```python
from build123d import *

# Parameters (mm, degrees)
F0_W      = 80
F0_H      = 30
F1_DEPTH  = 25
F3_DEPTH  = 20
F4_R      = 1.5
F5_DEPTH  = 1000
F3_FACE_W = 60.621056
F3_FACE_H = 22.732896
F6_DEPTH  = 25
F7_R      = 1.35
F7_R_2    = 1
F8_DEPTH  = 100000


with BuildPart() as f1:
    # F0 (on Front) → F1 (new body)
    with BuildSketch(Plane.XZ):
        with Locations((5.157232, 15)):
            Rectangle(F0_W, F0_H)
    extrude(amount=F1_DEPTH)

    # F2 (on face) → F3 (cut)
    with BuildSketch(Plane.XZ.offset(25)):
        Polygon((35.46776, 26.366448), (-25.153296, 26.366448), (5.157232, 15), align=None)
        Polygon((5.157232, 15), (-25.153296, 26.366448), (-25.153296, 3.633552), align=None)
        Polygon((35.46776, 26.366448), (5.157232, 15), (35.46776, 3.633552), align=None)
        Polygon((35.46776, 3.633552), (5.157232, 15), (-25.153296, 3.633552), align=None)
    extrude(amount=-F3_DEPTH, mode=Mode.SUBTRACT)

    # F4 (on face) → F5 (cut)
    with BuildSketch(Plane.YZ.offset(45.157232)):
        with Locations((-12.5, 15.157233)):
            Circle(F4_R)
    extrude(amount=-F5_DEPTH, mode=Mode.SUBTRACT)

    # F3_face (on face) → F6 (cut)
    with BuildSketch(Plane(origin=(5.157232, -5, 15), x_dir=(1, 0, 0), z_dir=(0, -1, 0))):
        Rectangle(F3_FACE_W, F3_FACE_H)
    extrude(amount=-F6_DEPTH, mode=Mode.SUBTRACT)

    # F7 (on face) → F8 (cut)
    with BuildSketch(Plane.XZ.offset(25)):
        with BuildLine():
            ThreePointArc((-29.95245, 20.807233), (-28.997856, 21.202639), (-28.60245, 22.157233))
            ThreePointArc((-28.60245, 22.157233), (-30.907045, 23.111827), (-29.95245, 20.807233))
        make_face()
        with Locations((-29.95245, 8.157233)):
            Circle(F7_R)
        with Locations((40.266914, 8.157233)):
            Circle(F7_R)
        with Locations((40.266914, 22.157233)):
            Circle(F7_R)
        with Locations((-12.661189, -18.048356)):
            Circle(F7_R_2)
    extrude(amount=-F8_DEPTH, mode=Mode.SUBTRACT)


solid = f1.part
```
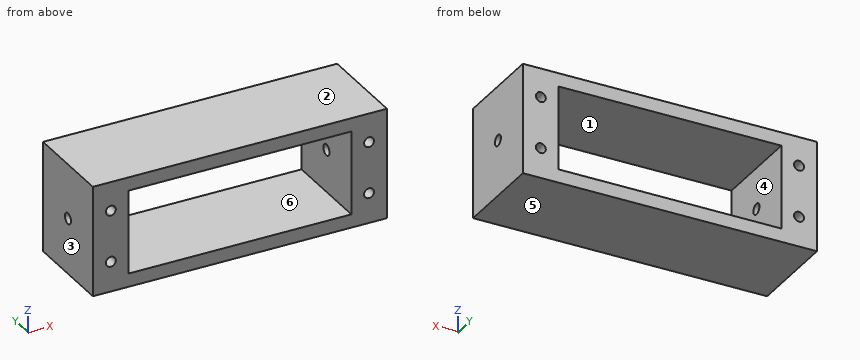
Can you work these out from the model? Positions are in its coordinate system, mm. Face numbers are marked on the shaded views. A direction names the side the tool comes from. Round coordinates to 2 decimals unless told otherwise and drop trailing zeros. Loops run counter-clockwise (first coordinate to the right, second up) from the corner with the lowest first, then second, coordinate; pieces in that order, holes last. Notation, with made-up numbers: M 22.25,88.5 L 48.25,88.5 A20 ccw 48.25,102.5 Z; hole C -22.5,47.5 d7. An arc over 180 degrees is marked long. Write item = value, one per line. Start each with the question number.
(1) I'm going to push a flat-ended pin straight in: P1, Ø2.5, axis at y = -12.5, z = 15.16, coming from the +X side. Where does the tip first touch, or does it pass through?
(2) If we mould it in two halves opening along X, with no side actions, what happens to the marked faces 1, 2, 3 and 4? For each: released by +X, released by -X, zero draft, split by the parting line, or undercut.
(3) Which directions (+Z, -Z, +X, -X, +Y, -Y) give clear straight access to the entire face, cutting with the end or side of a thin tool? Please do the marked faces 5 and 6.
(4) Suppose I cut it at C-C on x = 31.5. Write out the boundary of the cut face in (y, z).
(5) Suppose I cut it at A-A on z = 24.5. Write out the boundary of the cut face in (x, y), plus the area to 3 significant figures.
(6) I need wall thicknesses on line 1 along X through (y, z) = (-20.25, 8); line 2 along X through (y, z) = (-23, 5); line 3 along Z through (x, y) = (26, -22.5). Which ranges of each line are inside material? Lowest first, please.
(7) Suppose I cut it at B-B on y = -12.5. Write out the boundary of the cut face in (x, z), plus the area to 3 significant figures.
Answer block:
q1.P1 = through
q2.face_1 = undercut
q2.face_2 = zero draft
q2.face_3 = released by -X
q2.face_4 = undercut
q3.face_5 = -Z, +X, -X, +Y, -Y
q3.face_6 = +Y, -Y
q4.outline = M -25,0 L 0,0 L 0,3.63 L -25,3.63 Z; M -25,26.37 L 0,26.37 L 0,30 L -25,30 Z
q5.outline = M -34.84,-25 L -25.15,-25 L -25.15,0 L -34.84,0 Z; M 35.47,-25 L 45.16,-25 L 45.16,0 L 35.47,0 Z
q5.area = 484 mm²
q6.line_1 = -34.84 to -31.29, -28.61 to -25.15, 35.47 to 38.93, 41.61 to 45.16
q6.line_2 = -34.84 to -25.15, 35.47 to 45.16
q6.line_3 = 0 to 3.63, 26.37 to 30
q7.outline = M -34.84,0 L 45.16,0 L 45.16,13.66 L 35.47,13.66 L 35.47,3.63 L -25.15,3.63 L -25.15,13.66 L -34.84,13.66 Z; M -34.84,16.66 L -25.15,16.66 L -25.15,26.37 L 35.47,26.37 L 35.47,16.66 L 45.16,16.66 L 45.16,30 L -34.84,30 Z; hole C -29.95,8.16 d2.7; hole C -29.95,22.16 d2.7; hole C 40.27,8.16 d2.7; hole C 40.27,22.16 d2.7
q7.area = 941 mm²
